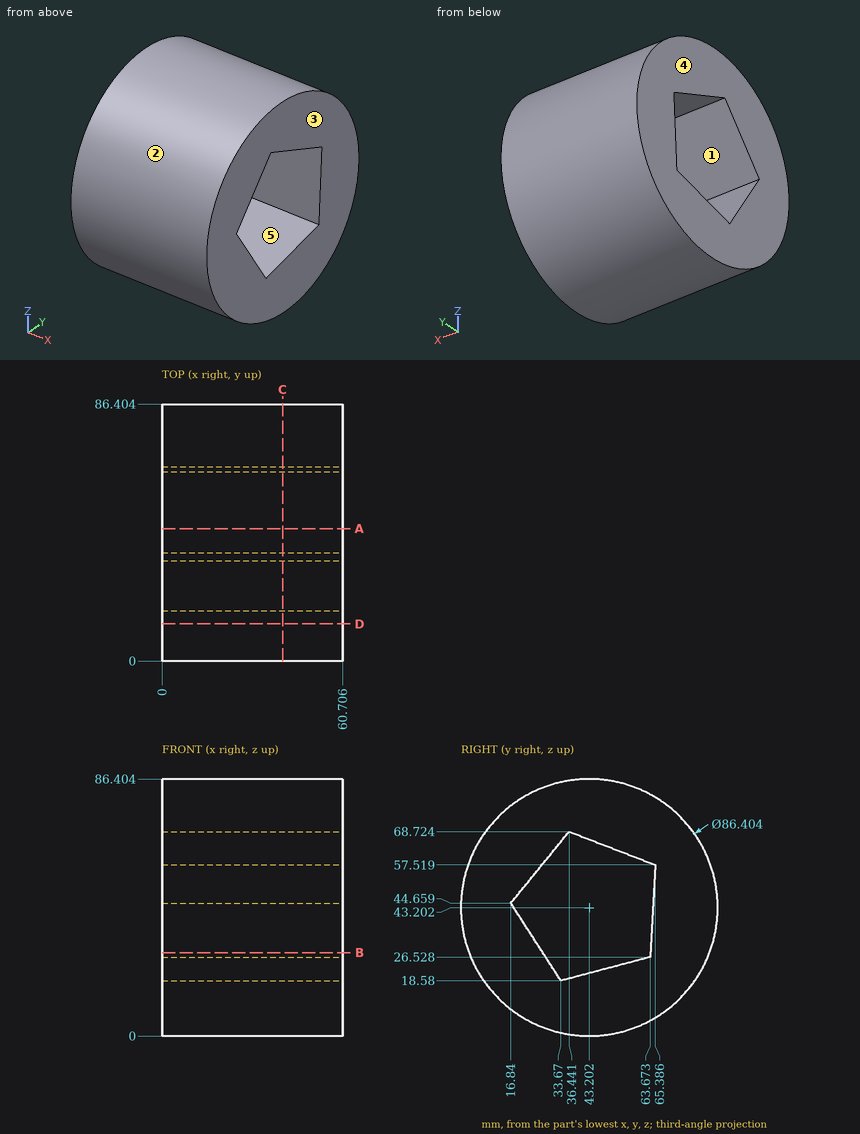
Study the drawing (mm; zero at the part's minimum x, y, z) and answer. A direction names the side the tool comes from. Coordinates: 2 decimals unless noted, no trailing zeros. Loops run counter-clockwise (first coordinate to the right, second up) from the corner with the lowest first, then second, coordinate; pieces in that order, holes last. Notation, with made-up numbers: (-11.5, 45) -> (-6.5, 45) arc R14 cw to (-6.5, 54) -> close; hole circle Ø11 at (55.5, 60.5). An arc over 180 degrees is marked (long way). Answer in a Markdown table with one row per item. Add a question column.
1. The part is cut by section D-D, the plane y = 12.5. Write down the section's boundary in (x, z).
2. Flat-ended cylindrical pins translate along their axes: P1, Ø10, axis at x = 40.5, z = 74.5, coming from the -Y side (1 decimal); P2, Ø2, axis at x = 43, z = 48.5, coming from the +Y side; P3, Ø1.5, axis at x = 44.5, z = 25, coming from the -Y side; P4, Ø10, axis at y = 32, z = 52.5, coming from the +X side. Find the tip coordinate at first contact, or state that the pin passes through.
3. For the marked faces 4 and 5, determine the directions among +Z, -Z, +X, -X, +Y, -Y from which every point of the face is accessible in a straight line to the end or side of a thin tool.
4. The part is cut by section A-A, the plane y = 44.5. Write down the section's boundary in (x, z) (1 decimal).
5. Determine the mould class of the marked faces 1, 2 and 3 for opening direction Z: +Z half, -Z half, draft (parallel to the pull), parting line (faces both ways), or undercut.
6. The part is cut by section C-C, the plane x = 40.5. Write down the section's boundary in (y, z) (1 decimal).
7. Consider line 1 (Z direction, x = 37, y = 51) (1 decimal); line 2 (Z direction, x = 57.5, y = 24.5) (1 decimal); line 3 (Y direction, x = 42.5, z = 45) (1 decimal). Determine where each line is inside the solid, lowest interval first. Write a range as [from, to].
8. The part is cut by section B-B, the plane z = 28. Write down the section's boundary in (x, y) (1 decimal), then the cut area to 3 significant figures.
Answer below:
| question | item | result |
|---|---|---|
| 1 | outline | (0, 12.81) -> (60.71, 12.81) -> (60.71, 73.6) -> (0, 73.6) -> close |
| 2 | P1 | y = 8.9 |
| 2 | P2 | y = 86.19 |
| 2 | P3 | y = 3.68 |
| 2 | P4 | through |
| 3 | face 4 | +Z, -Z, -X, +Y, -Y |
| 3 | face 5 | +X, -X |
| 4 | outline | (0, 0) -> (60.7, 0) -> (60.7, 21.4) -> (0, 21.4) -> close; (0, 65.6) -> (60.7, 65.6) -> (60.7, 86.4) -> (0, 86.4) -> close |
| 5 | face 1 | undercut |
| 5 | face 2 | parting line |
| 5 | face 3 | draft |
| 6 | outline | circle Ø86.4 at (43.2, 43.2); hole (16.8, 44.7) -> (33.7, 18.6) -> (63.7, 26.5) -> (65.4, 57.5) -> (36.4, 68.7) -> close |
| 7 | line 1 | [0.7, 23.2], [63.1, 85.7] |
| 7 | line 2 | [4.3, 32.8], [54.1, 82.1] |
| 7 | line 3 | [0, 17.1], [64.7, 86.4] |
| 8 | outline | (0, 2.8) -> (60.7, 2.8) -> (60.7, 27.6) -> (0, 27.6) -> close; (0, 63.8) -> (60.7, 63.8) -> (60.7, 83.6) -> (0, 83.6) -> close |
| 8 | area | 2,710 mm2 |
